Read the model definition and answer for the solid it produces. Units are mm, in the model's axes. Face numbers are marked on the shaded views. A direction names the side the tool comes from. Give positions to 0.01 mm unless a question says otherwise; leave off trailing zeros. Write each loop counter-clockwise with the first axis right and the second up, starting at its lowest first coordinate (ties: lowest second). Pieces come first, ordered by that corner, then holes. Notation, with made-up numbers: M 21,57 L 57,57 A16 cw 57,73 Z; hole C -7.5,7.5 d4. An arc over 180 degrees is marked long. Answer as CSV lines item,"result". Start each with the question number.
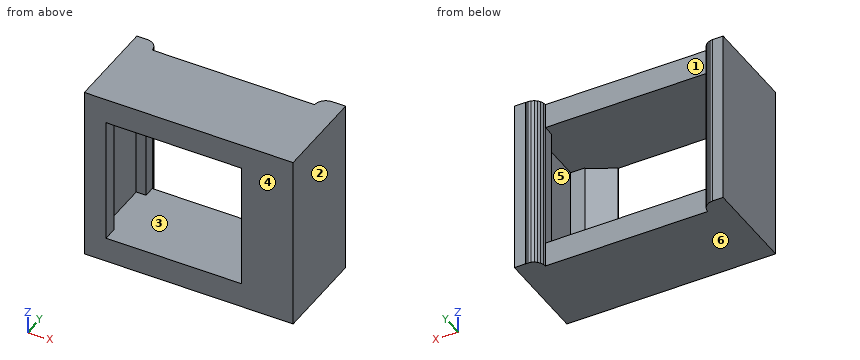
Autodesk Fusion 360 part; units mm, degrees
sketch "keystone-side" plane through (0, 0, 0) normal (0, 0, 1) x (1, 0, 0)
  line L0 (0.3425, -57.6967) -> (0.6681, -57.5618)
  line L1 (-19.7725, -68.7658) -> (-19.7725, -67.0158)
  line L2 (1.2775, -57.55) -> (1.2775, -57.5158)
  line L3 (-19.7725, -58.8658) -> (-0.3325, -58.8658)
  line L4 (-0.4364, -67.1264) -> (-3.5225, -68.7192)
  line L5 (2.6275, -57.5158) -> (2.6275, -68.7658)
  line L6 (1.0175, -57.5158) -> (1.2775, -57.55)
  line L7 (-3.5225, -68.7658) -> (-19.7725, -68.7658)
  line L8 (0.6681, -57.5618) -> (1.0175, -57.5158)
  line L9 (-20.9425, -67.0158) -> (-20.9425, -60.2158)
  line L10 (1.2775, -57.5158) -> (2.6275, -57.5158)
  line L11 (-19.9533, -58.1908) -> (-19.8185, -58.5164)
  line L12 (-19.7725, -58.8658) -> (-0.3325, -58.8658)
  line L13 (-20.9425, -60.2158) -> (-19.7725, -60.2158)
  line L14 (0.0629, -57.9112) -> (0.3425, -57.6967)
  line L15 (-0.3325, -58.8658) -> (-0.3325, -60.2158)
  line L16 (-0.1516, -58.1908) -> (0.0629, -57.9112)
  line L17 (-19.7725, -67.0158) -> (-20.9425, -67.0158)
  line L18 (2.6275, -68.7658) -> (-22.3725, -68.7658)
  line L19 (-20.7731, -57.5618) -> (-20.4475, -57.6967)
  line L20 (-0.3325, -60.2158) -> (1.1975, -60.2158)
  line L21 (-20.4475, -57.6967) -> (-20.1679, -57.9112)
  line L22 (-19.7725, -60.2158) -> (-19.7725, -58.8658)
  line L23 (1.1975, -67.0158) -> (-0.4934, -67.0158)
  line L24 (-22.3725, -57.5158) -> (-21.1225, -57.5158)
  line L25 (-22.3725, -68.7658) -> (-22.3725, -57.5158)
  line L26 (-21.1225, -57.5158) -> (-20.7731, -57.5618)
  line L27 (-0.4934, -67.0158) -> (-0.4364, -67.1264)
  line L28 (-20.1679, -57.9112) -> (-19.9533, -58.1908)
  line L29 (-19.8185, -58.5164) -> (-19.7725, -58.8658)
  line L30 (-0.2865, -58.5164) -> (-0.1516, -58.1908)
  line L31 (-3.5225, -68.7192) -> (-3.5225, -68.7658)
  line L32 (-0.3325, -58.8658) -> (-0.2865, -58.5164)
  line L33 (1.1975, -60.2158) -> (1.1975, -67.0158)
  line L34 (-19.7725, -60.2158) -> (-0.3325, -60.2158)
extrude "Extrude1" add sketch "keystone-side" along normal blind 3
extrude "Extrude2" add sketch "keystone-side" against normal blind 18.1
extrude "Extrude3" cut sketch "keystone-side" against normal blind 15.1 contours L3 L12 L15 L22 L34 | L1 L4 L7 L9 L13 L17 L18 L20 L23 L27 L31 L33 L34
1. Find section C-C on x = -8.5. Determine the outline of the cut face in (y, z), then the cut area to 3 significant figures.
2. Determine the mould class of the marked faces 4, 5 and 6 for opening direction Y: +Y half, -Y half, draft (parallel to the pull), parting line (faces both ways), or undercut.
3. Given pin 1 (2.5 mm diameter, centred on x = -14, z = -17, fed in from +Y); pin 2 (0.9 mm diameter, centred on x = -20.5, z = -9, fed in from +Y); pin 3 (6 mm diameter, centred on x = -9, z = -5.5, fed in from -Y), each flat-ended and moving along its own axis, determine where each tip first touches the part or whether it passes through.
4. Find the intervals of material crossed by line 1 (Z direction, x = -1.25, y = -62.5); line 2 (X direction, y = -58.5, z = -15.75); line 3 (X direction, y = -63.75, z = -8), in increasing order. Write a range as [from, to].
5. Find section A-A on y = -63.5. Determine the outline of the cut face in (x, z), then the cut area to 3 significant figures.
6. For the marked faces 1, 2 and 3, determine the directions among +Z, -Z, +X, -X, +Y, -Y from which every point of the face is accessible in a straight line to the end or side of a thin tool.
Computed:
1,outline,"M -68.77,-18.1 L -58.87,-18.1 L -58.87,-15.1 L -68.77,-15.1 Z; M -68.77,0 L -58.87,0 L -58.87,3 L -68.77,3 Z"
1,area,"59.4 mm^2"
2,face 4,"-Y half"
2,face 5,"undercut"
2,face 6,"draft"
3,pin 1,"stops at y = -58.87"
3,pin 2,"stops at y = -57.54"
3,pin 3,"passes through"
4,line 1,"z = [-18.1, -15.1], [0, 3]"
4,line 2,"x = [-22.37, -19.83], [-0.28, 2.63]"
4,line 3,"x = [-22.37, -20.94], [1.2, 2.63]"
5,outline,"M -22.37,-18.1 L 2.63,-18.1 L 2.63,3 L -22.37,3 Z; hole M -20.94,-15.1 L 1.2,-15.1 L 1.2,0 L -20.94,0 Z"
5,area,"193 mm^2"
6,face 1,"+Z, -Z, +Y"
6,face 2,"+Z, -Z, +X, +Y, -Y"
6,face 3,"none"
